Here's how the part is built. I have some questions about the finished solid (model axes, mm). Face numbers are marked on the shaded views. Give positions to 0.01 mm unless a question says otherwise; leave off trailing zeros. Write each loop counter-clockwise with the first axis right and the second up, starting at its lowest first coordinate (ties: lowest second). Pieces come first, ordered by that corner, then holes. Notation, with made-up numbers: (35.25, 81.5) -> (40.25, 81.5) arc R19 ccw to (40.25, 111.5) -> close; hole circle Ø10 at (26, 83). An arc over 180 degrees is marked (long way). Return JSON: item names as keys, results as strings.
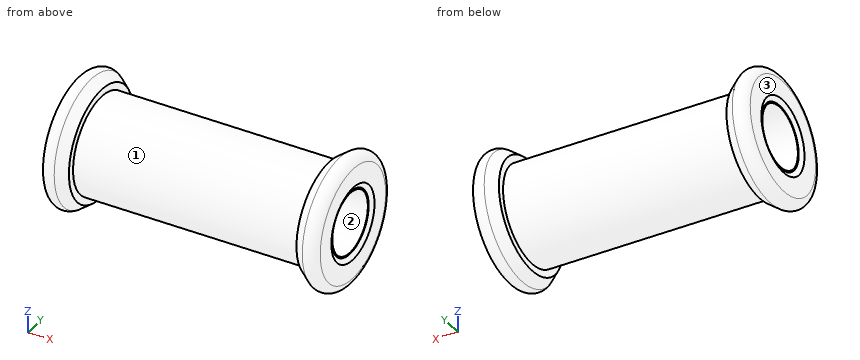
from build123d import *

# Parameters (mm, degrees)
SKETCH4_R          = 2.15
CUT_EXTRUDE1_DEPTH = 28


with BuildPart() as part:
    # Sketch1 → Revolve1 (revolve)
    with BuildSketch(Plane.XY):
        with BuildLine():
            Line((-37.045023651, 0), (-18.045023651, 0))
            Line((-18.045023651, 0), (-18.045023651, 2.25))
            Line((-18.045023651, 2.25), (-17.846575332, 2.610383943))
            Line((-17.846575332, 2.610383943), (-17.846575332, 3.959600078))
            ThreePointArc((-17.846575332, 3.959600078), (-18.183709968, 4.505741021), (-18.823024722, 4.449116479))
            Line((-18.823024722, 4.449116479), (-19.545023651, 3.91))
            Line((-19.545023651, 3.91), (-19.545023651, 3.41))
            Line((-19.545023651, 3.41), (-35.545023651, 3.41))
            Line((-35.545023651, 3.41), (-35.545023651, 3.91))
            Line((-35.545023651, 3.91), (-36.267022579, 4.449116479))
            ThreePointArc((-36.267022579, 4.449116479), (-36.906337333, 4.505741021), (-37.24347197, 3.959600078))
            Line((-37.24347197, 3.959600078), (-37.24347197, 2.610383943))
            Line((-37.24347197, 2.610383943), (-37.045023651, 2.25))
            Line((-37.045023651, 2.25), (-37.045023651, 0))
        make_face()
    revolve(axis=Axis((-9.250519902, 0, 0), (-1, 0, 0)))

    # Sketch4 → Cut-Extrude1 (cut)
    with BuildSketch(Plane(origin=(-18.045023651, 0, 0), x_dir=(0, 0, -1), z_dir=(1, 0, 0))):
        with Locations(Location((0, 0, 0), (0, 0, 90))):
            Circle(SKETCH4_R)
    extrude(amount=-CUT_EXTRUDE1_DEPTH, mode=Mode.SUBTRACT)


solid = part.part
1. Suppose I cut it at D-D, the plane x = -36. List the corners of the cut face in (y, z) for me, and give its area (3 significant figures).
Taken from the geometry:
{"outline": "circle Ø8.5 at (0, 0); hole circle Ø4.3 at (0, 0)", "area": "42.2 mm²"}
2. If we mould it in two halves opening along X, with no side actions, what happens to the marked faces 1, 2 and 3? For each: released by +X, released by -X, zero draft, split by the parting line, or undercut.
Taken from the geometry:
{"face 1": "undercut", "face 2": "zero draft", "face 3": "released by -X"}
3. Suppose I cut it at A-A, the plane y = 0. List the corners of the cut face in (x, z) for me, and give its area (3 significant figures).
Taken from the geometry:
{"outline": "(-37.24, -3.96) arc R0.61 ccw to (-36.27, -4.45) -> (-35.55, -3.91) -> (-35.55, -3.41) -> (-19.55, -3.41) -> (-19.55, -3.91) -> (-18.82, -4.45) arc R0.61 ccw to (-17.85, -3.96) -> (-17.85, -2.61) -> (-18.05, -2.25) -> (-18.05, -2.15) -> (-37.05, -2.15) -> (-37.05, -2.25) -> (-37.24, -2.61) -> close; (-37.24, 2.61) -> (-37.05, 2.25) -> (-37.05, 2.15) -> (-18.05, 2.15) -> (-18.05, 2.25) -> (-17.85, 2.61) -> (-17.85, 3.96) arc R0.61 ccw to (-18.82, 4.45) -> (-19.55, 3.91) -> (-19.55, 3.41) -> (-35.55, 3.41) -> (-35.55, 3.91) -> (-36.27, 4.45) arc R0.61 ccw to (-37.24, 3.96) -> close", "area": "55.0 mm²"}
4. Suppose I cut it at C-C, the plane x = -31. List the corners of the cut face in (y, z) for me.
Taken from the geometry:
{"outline": "circle Ø6.82 at (0, 0); hole circle Ø4.3 at (0, 0)"}
5. For pin 1 Ø1.5 at (x, z) = (-31, -2) entering from -Y; pin 2 Ø1.5 at (x, y) = (-25, -1.5) entering from -Z; pin 3 Ø1 at (x, y) = (-26, 2) entering from +Z, each with a flat end and sliding along its axis, tell me the tip position at first contact or that it passes through.
Taken from the geometry:
{"pin 1": "stops at y = -3.17", "pin 2": "stops at z = -3.33", "pin 3": "stops at z = 3.06"}
6. If I drill on line 1 (Z direction, x = -28, y = 0); line 2 (X direction, y = -2.5, z = -2.75); line 3 (Z direction, x = -30.75, y = -1.5), over which ranges is the centre line in solid material (lowest first)? Write a range as [from, to].
Taken from the geometry:
{"line 1": "z = [-3.41, -2.15], [2.15, 3.41]", "line 2": "x = [-37.24, -35.55], [-19.55, -17.85]", "line 3": "z = [-3.06, -1.54], [1.54, 3.06]"}
